Could you check a few things on this model? Use its own coordinates, in mm. Face numbers are marked on the shaded views. Round coordinates to 2 decimals unless told otherwise and drop trailing zeros. Write each loop counter-clockwise with the first axis right and the second up, starting at its lowest first coordinate (ties: lowest second). Pieces come first, ordered by that corner, then holes. Notation, with made-up numbers: (66.25, 24.5) -> (123.25, 24.5) arc R10 ccw to (123.25, 32.5) -> close; hole circle Ø2 at (30.25, 44.5). An arc over 180 degrees is marked (long way). Answer in a Markdown table with one row per item.
Autodesk Inventor part; units mm, degrees
ref_plane "YZ Plane" through (0, 0, 0) normal (1, 0, 0) x (0, 1, 0)
ref_plane "XZ Plane" through (0, 0, 0) normal (0, 1, 0) x (-1, 0, 0)
ref_plane "XY Plane" through (0, 0, 0) normal (0, 0, 1) x (1, 0, 0)
sketch "Sketch1" plane through (0, 0, 0) normal (0, 1, 0) x (-1, 0, 0)
  line L0 (14.234, 0) -> (-14.234, 0)
  line L1 (14.234, 0) -> (14.234, -16)
  line L2 (14.234, -16) -> (-14.234, -16)
  line L3 (-14.234, 0) -> (-14.234, -16)
  line L4 (16.234, 0) -> (16.234, -8.975)
  line L5 (16.234, -8.975) -> (14.234, -8.975)
  line L6 (16.234, 0) -> (14.234, 0)
  line L7 (0, 0) -> (0, -16) construction
  line L8 (-16.234, 0) -> (-16.234, -8.975)
  line L9 (-16.234, -8.975) -> (-14.234, -8.975)
  line L10 (-16.234, 0) -> (-14.234, 0)
  point P0 (-14.234, -8.975)
  dimension "d0" = 28.468
  dimension "d1" = 16
  dimension "d2" = 8.975
  dimension "d3" = 2
  dimension "d52" = 16
  dimension "d53" = 14.234
  dimension "d54" = 14.234
  dimension "d55" = 32.468
revolve "Revolution1" add sketch "Sketch1" angle 360 about axis through (-14.234, 0, 0) along (1, 0, 0)
sketch "Sketch3" plane through (14.234, 0, 0) normal (1, 0, 0) x (0, 0, -1)
  line L0 (0, 0) -> (0, 21.0687)
  circle A0 centre (0, 0) radius 12
  line L1 (0, 0) -> (15.1968, 15.1968)
  circle A1 centre (8.4853, 8.4853) radius 1.5075
  dimension "d12" = 24
  dimension "d13" = 45
  dimension "d14" = 3.015
extrude "Extrusion1" cut sketch "Sketch3" against normal through all contours A1 A0 L1 | L1 A0 A1 | A1 L1 A0 | L1 A1 A0
thread "Thread1"
sketch "Sketch5" plane through (16.234, 0, 0) normal (1, 0, 0) x (0, 0, -1)
  circle A0 centre (0, 0) radius 8.975
  point P0 (0, 0)
hole "Hole3" at (16.234, 0, 0) direction (-1, 0, 0) diameter 15 end through all
pattern_circular "Circular Pattern3" count 4 over 360 about axis through (-39.4631, 0, 0) along (1, 0, 0) of "Extrusion1"
properties part number "shaft" material "Stainless Steel"
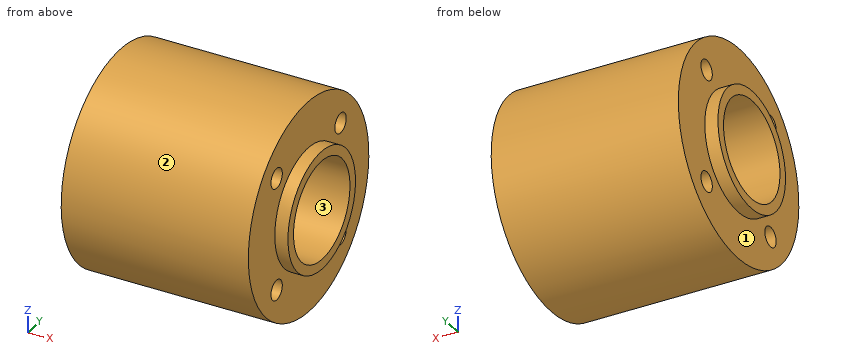
1) Imagine slicing it at D-D, the plane y = -14. Please give me the cut outline in (x, z), plus the area to 3 significant figures.
Findings:
| item | result |
|---|---|
| outline | (-14.23, -7.75) -> (14.23, -7.75) -> (14.23, 7.75) -> (-14.23, 7.75) -> close |
| area | 441 mm^2 |
2) Please list where these lines run through material, in increasing order: line 1 (X direction, y = 9, z = -1); line 2 (Y direction, x = -8, z = -9); line 3 (Z direction, x = 0.5, y = 5).
Findings:
| item | result |
|---|---|
| line 1 | x = -14.23 to 14.23 |
| line 2 | y = -13.23 to -9.9, -7.07 to 7.07, 9.9 to 13.23 |
| line 3 | z = -15.2 to -5.59, 5.59 to 15.2 |
3) Imagine slicing it at C-C, the plane x = 7.5. Please give me the cut outline in (y, z) (1 decimal).
Findings:
| item | result |
|---|---|
| outline | circle Ø32 at (0, 0); hole circle Ø3 at (-8.5, -8.5); hole circle Ø3 at (-8.5, 8.5); hole circle Ø15 at (0, 0); hole circle Ø3 at (8.5, -8.5); hole circle Ø3 at (8.5, 8.5) |
4) For pin 1 (17 mm diameter, centred on y = 0, z = 0, fed in from -X); pin 2 (4 mm diameter, centred on x = -1.5, y = 6.5, fed in from -Z); pin 3 (2 mm diameter, centred on x = 3.5, y = 8, fed in from -Z); pin 4 (10 mm diameter, centred on x = 0, z = -5.5, fed in from -Y), each with a flat end and sliding along its axis, tell me the tip position at first contact or that it passes through.
Findings:
| item | result |
|---|---|
| pin 1 | stops at x = -16.23 |
| pin 2 | stops at z = -15.35 |
| pin 3 | stops at z = -14.39 |
| pin 4 | stops at y = -15.99 |
5) Thinking about a two-plate mould opening in Y: for the marked faces 1, 2 and 3, which applies, +Y half, -Y half, draft (parallel to the pull), parting line (faces both ways), or undercut?
Findings:
| item | result |
|---|---|
| face 1 | draft |
| face 2 | parting line |
| face 3 | undercut |
6) Imagine slicing it at A-A, the plane z = 0. Please give me the cut outline in (x, y) (3 decimals).
Findings:
| item | result |
|---|---|
| outline | (-16.234, -8.975) -> (-14.234, -8.975) -> (-14.234, -16) -> (14.234, -16) -> (14.234, -8.975) -> (16.234, -8.975) -> (16.234, -7.5) -> (-16.234, -7.5) -> close; (-16.234, 7.5) -> (16.234, 7.5) -> (16.234, 8.975) -> (14.234, 8.975) -> (14.234, 16) -> (-14.234, 16) -> (-14.234, 8.975) -> (-16.234, 8.975) -> close |
